Source: CAD feature listing. Evaluate the final solid. Frame: model axes, mm. A direction names the side the tool comes from. Coordinates: 2 decimals unless noted, no trailing zeros. Loops run counter-clockwise (first coordinate to the right, second up) from the corner with the lowest first, then second, coordinate; pieces in that order, holes last. Notation, with made-up numbers: (0, 70) -> (44, 70) arc R13 ccw to (44, 93) -> close; hole circle Ø11 at (-26.5, 77.5). An arc over 180 degrees is marked (long way). Answer as CSV lines item,"result".
from build123d import *

# Parameters (mm, degrees)
F1_DEPTH = 38.1
F3_DEPTH = 12.7


with BuildPart() as f1:
    # F0 (on Right) → F1 (new body)
    with BuildSketch(Plane.YZ):
        Polygon((0, 6.35), (0, 0), (25.4, 0), (25.4, 31.901197), (19.05, 31.901197), align=None)
    extrude(amount=F1_DEPTH)

    # F2 (on face) → F3 (join)
    with BuildSketch(Plane(origin=(0, 0, 0), x_dir=(0, -1, 0), z_dir=(-1, 0, 0))):
        Polygon((0, 31.901197), (-19.05, 31.901197), (0, 6.35), align=None)
    extrude(amount=-F3_DEPTH)


solid = f1.part
(1) Pin query (flat end, axial travel): pin 1 Ø5 at (x, y) = (31.5, 16.5) entering from +Z; pin 2 Ø8 at (x, y) = (29.5, 9) entering from +Z; pin 3 Ø1.5 at (x, z) = (21.5, 18) entering from -Y; pin 4 Ø1 at (y, z) = (6, 25) entering from -X. Return the tip coordinate at first contact, or that it passes through.
Computed values:
pin 1,"z = 31.83"
pin 2,"z = 23.79"
pin 3,"y = 8.13"
pin 4,"x = 0"
(2) Material intervals for L1, parallel to X at y = 6.25, z = 20; L2, parallel to Z at x = 28.5, y = 12.25; L3, parallel to Y at x = 13, z = 10, sorted ascending. Write a range as [from, to].
Computed values:
L1,"[0, 12.7]"
L2,"[0, 22.78]"
L3,"[2.72, 25.4]"
(3) Cut plane A-A (x = 16). Return the cut outline in (y, z).
Computed values:
outline,"(0, 0) -> (25.4, 0) -> (25.4, 31.9) -> (19.05, 31.9) -> (0, 6.35) -> close"
(4) Cut plane C-C (z = 25). Return the cut outline in (x, y), then the cut area to 3 significant figures.
Computed values:
outline,"(0, 0) -> (12.7, 0) -> (12.7, 13.9) -> (38.1, 13.9) -> (38.1, 25.4) -> (0, 25.4) -> close"
area,"615 mm^2"
(5) Access query for faces 1 (the flat face through (10, 15, 31.901)), 2 (the flat face through (25.222, 9.658, 19.304)). Directions: +Z, -Z, +X, -X, +Y, -Y. A direction counts if a zero-diameter tool reaches every point of the face in a straight line with its end or side. Return the directions, or none.
Computed values:
face 1,"+Z, +X, -X, +Y, -Y"
face 2,"+Z, +X, -Y"
(6) Cut plane B-B (y = 7.25). Return the cut outline in (x, z).
Computed values:
outline,"(0, 0) -> (38.1, 0) -> (38.1, 16.07) -> (12.7, 16.07) -> (12.7, 31.9) -> (0, 31.9) -> close"
